from build123d import *

# Parameters (mm, degrees)
F0_W     = 40
F0_H     = 25
F1_DEPTH = 2
F2_W     = 2
F2_H     = 15
F3_DEPTH = 2
F5_DEPTH = 2.001


# Not quite as in the source:
# - a pattern or mirror of a feature is missing from the dataset's text; its kind, count and spacing are read off the source's solid


with BuildPart() as f1:
    # F0 (on Top) → F1 (new body)
    with BuildSketch(Plane.XY):
        Rectangle(F0_W, F0_H)
    extrude(amount=F1_DEPTH)

    # F2 (on Top) → F3 (join)
    with BuildSketch(Plane.XY):
        with Locations((-21, 0)):
            Rectangle(F2_W, F2_H)
    f3 = extrude(amount=F3_DEPTH)

    # F3_copies: F3 across plane
    add(f3.mirror(Plane(origin=(0, 0, 0), x_dir=(0, 0, 1), z_dir=(1, 0, 0))))

    # F4 (on face) → F5 (cut, through all)
    with BuildSketch(Plane.XY.offset(2)):
        with BuildLine():
            ThreePointArc((-13.75, 5), (-15, 6.25), (-16.25, 5))
            Line((-16.25, 5), (-16.25, -5))
            ThreePointArc((-16.25, -5), (-15, -6.25), (-13.75, -5))
            Line((-13.75, -5), (-13.75, 5))
        make_face()
    f5 = extrude(amount=-F5_DEPTH, mode=Mode.SUBTRACT)

    # F5_copies: F5 across plane
    add(f5.mirror(Plane(origin=(0, 0, 0), x_dir=(0, 0, 1), z_dir=(1, 0, 0))), mode=Mode.SUBTRACT)


solid = f1.part
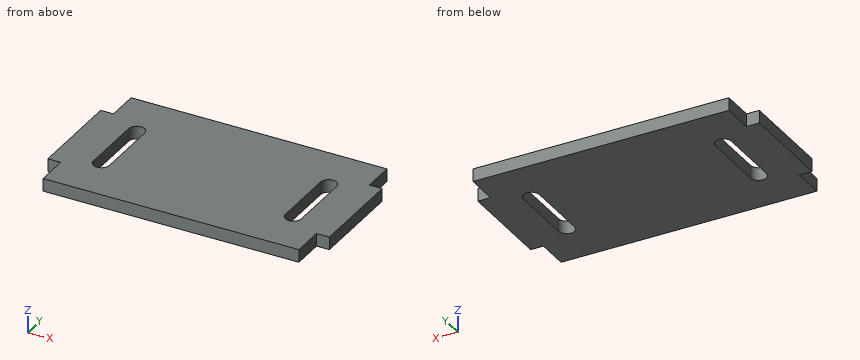
CAD build for the part. Positions are in the model's coordinates, mm. Coordinates: 2 decimals unless noted, no trailing zeros. Order: outer loops, then holes, each group sorted by start corner. A loop starts at its lowest first (then second) coordinate and runs counter-clockwise, first axis right, second up. Notation, with made-up numbers: (15, -13.75) -> (62, -13.75) arc R8 cw to (62, -9.75) -> close; hole circle Ø5 at (-20, -34.5). An arc over 180 degrees is marked (long way). Answer in a Markdown table with one row per item.
1) Drill centre lines: line 1 (X direction, y = 0.25, z = 1.65); line 2 (X direction, y = 8.75, z = 0.9); line 3 (Y direction, x = -15.5, z = 0.25). Where is each one in solid material? Low to high.
Check values:
| item | result |
|---|---|
| line 1 | -22 to -16.25, -13.75 to 13.75, 16.25 to 22 |
| line 2 | -20 to 20 |
| line 3 | -12.5 to -6.15, 6.15 to 12.5 |
2) Band-saw the part on C-C (y = 5.5). List the corners of the cut face in (x, z).
Check values:
| item | result |
|---|---|
| outline | (-22, 0) -> (-16.15, 0) -> (-16.15, 2) -> (-22, 2) -> close; (-13.85, 0) -> (13.85, 0) -> (13.85, 2) -> (-13.85, 2) -> close; (16.15, 0) -> (22, 0) -> (22, 2) -> (16.15, 2) -> close |
3) Band-saw the part on B-B (z = 1.25). List the corners of the cut face in (x, y), and give its area (3 significant figures).
Check values:
| item | result |
|---|---|
| outline | (-22, -7.5) -> (-20, -7.5) -> (-20, -12.5) -> (20, -12.5) -> (20, -7.5) -> (22, -7.5) -> (22, 7.5) -> (20, 7.5) -> (20, 12.5) -> (-20, 12.5) -> (-20, 7.5) -> (-22, 7.5) -> close; hole (-16.25, -5) arc R1.25 ccw to (-13.75, -5) -> (-13.75, 5) arc R1.25 ccw to (-16.25, 5) -> close; hole (13.75, -5) arc R1.25 ccw to (16.25, -5) -> (16.25, 5) arc R1.25 ccw to (13.75, 5) -> close |
| area | 1,000 mm2 |
4) Band-saw the part on A-A (x = -15). List the corners of the cut face in (y, z).
Check values:
| item | result |
|---|---|
| outline | (-12.5, 0) -> (-6.25, 0) -> (-6.25, 2) -> (-12.5, 2) -> close; (6.25, 0) -> (12.5, 0) -> (12.5, 2) -> (6.25, 2) -> close |
5) Flat gauge pins, fed straight in: P1, Ø1, axis at x = -21, z = 1.5, coming from the +Y side; P2, Ø0.6, axis at y = -9, z = 1.5, coming from the -X side; P3, Ø1, axis at x = -21.5, z = 1.5, coming from the -Y side. Where does each tip first touch, or does it go through?
Check values:
| item | result |
|---|---|
| P1 | y = 7.5 |
| P2 | x = -20 |
| P3 | y = -7.5 |
6) Band-saw the part on D-D (y = -10.25). List the corners of the cut face in (x, z), and give its area (3 significant figures).
Check values:
| item | result |
|---|---|
| outline | (-20, 0) -> (20, 0) -> (20, 2) -> (-20, 2) -> close |
| area | 80.0 mm2 |
